Geometry: see drawing. Coordinates: mm, zero at the bounding-box minimum. Coordinates: 2 decimals unless noted, no trailing zeros. Write each loop counter-clockwise with the first axis right and the second up, starting at its lowest first coordinate (ties: lowest second). Pieces come first, ordered by that corner, then holes.
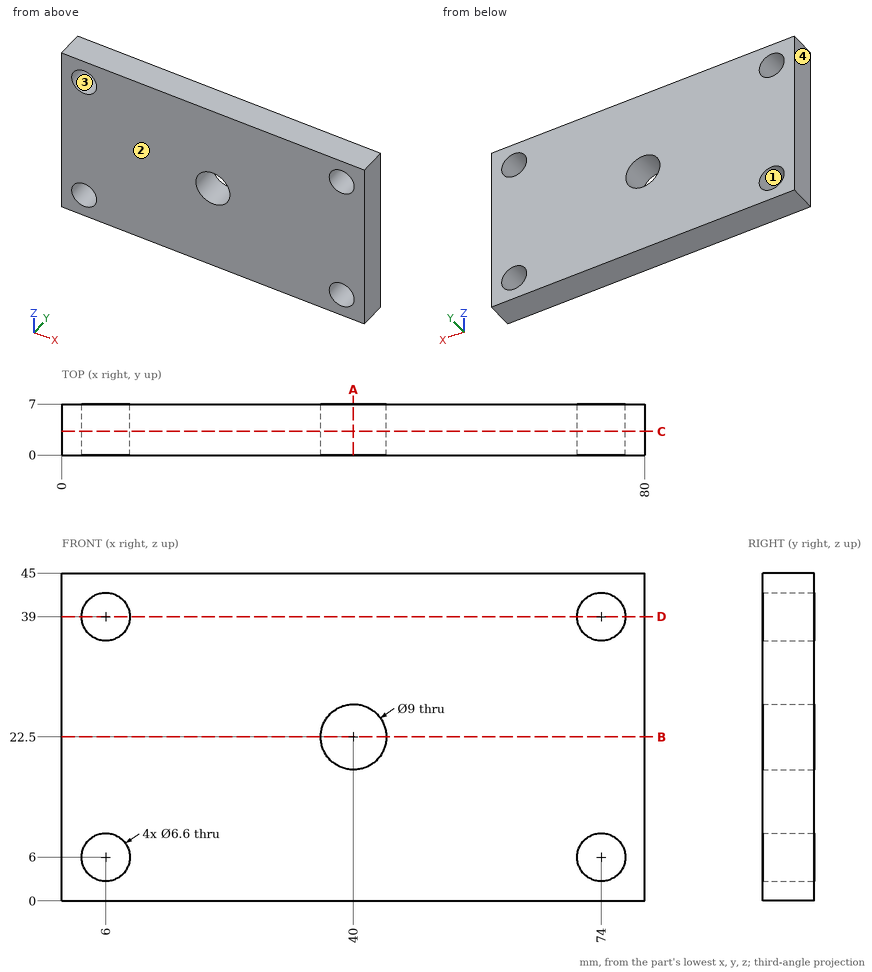
Item 1: Section B-B, the plane z = 22.5. Output: boundary loops of the cut face in (x, y).
Derived:
outline: (0, 0) - (35.5, 0) - (35.5, 7) - (0, 7) - close; (44.5, 0) - (80, 0) - (80, 7) - (44.5, 7) - close
Item 2: Section D-D, the plane z = 39. Output: boundary loops of the cut face in (x, y).
Derived:
outline: (0, 0) - (2.7, 0) - (2.7, 7) - (0, 7) - close; (9.3, 0) - (70.7, 0) - (70.7, 7) - (9.3, 7) - close; (77.3, 0) - (80, 0) - (80, 7) - (77.3, 7) - close
Item 3: Section A-A, the plane x = 40. Output: boundary loops of the cut face in (y, z), plus the area to 3 significant figures.
Derived:
outline: (0, 0) - (7, 0) - (7, 18) - (0, 18) - close; (0, 27) - (7, 27) - (7, 45) - (0, 45) - close
area: 252 mm2
Item 4: Section C-C, the plane y = 3.25. Output: boundary loops of the cut face in (x, z).
Derived:
outline: (0, 0) - (80, 0) - (80, 45) - (0, 45) - close; hole circle Ø6.6 at (6, 6); hole circle Ø6.6 at (6, 39); hole circle Ø9 at (40, 22.5); hole circle Ø6.6 at (74, 6); hole circle Ø6.6 at (74, 39)
Item 5: Pull-direction query (X, two-part tool) for the marked faces 1, 2, 3 and 4; classes: released by +X, released by -X, zero draft, split by the parting line, or undercut.
Derived:
face 1: undercut
face 2: zero draft
face 3: undercut
face 4: released by -X
Item 6: Material intervals for probe 1 along Z at (x, y) = (6, 1.75); probe 2 along X at (y, z) = (4.5, 6.5); probe 3 along X at (y, z) = (3.25, 8), sorted ascending.
Derived:
probe 1: z = 0 to 2.7, 9.3 to 35.7, 42.3 to 45
probe 2: x = 0 to 2.74, 9.26 to 70.74, 77.26 to 80
probe 3: x = 0 to 3.38, 8.62 to 71.38, 76.62 to 80
